from build123d import *

# Parameters (mm, degrees)
F0_W     = 112
F0_H     = 120
F1_DEPTH = 20
F2_DEPTH = 60
F3_SIZE2 = 34.641006
F3_SIZE  = 59.99999
F4_SIZE2 = 34.641006
F4_SIZE  = 59.99999
F5_R     = 20
F7_R     = 30
F8_R     = 10


# Not quite as in the source:
# - a fillet or chamfer is up to 0.001 mm smaller than in the source, because OpenCascade refuses the exact size


with BuildPart() as f1:
    # F0 (on Top) → F1 (new body)
    with BuildSketch(Plane.XY):
        with Locations((0.0172033906, -34.0157587473)):
            Rectangle(F0_W, F0_H)
    extrude(amount=F1_DEPTH)


with BuildPart() as f2:
    # F2 (new): a face of the model
    f2_faces = [f1.part.faces().sort_by_distance(p)[0] for p in [
        (0.0172033906, -34.0157587473, 20),
    ]]
    extrude(f2_faces, amount=F2_DEPTH)

    # F3 (size 60 and 34.6410161514 in the source; OpenCascade refuses exactly that, so slightly less here)
    f3_edges = [f2.edges().sort_by_distance(p)[0] for p in [
        (56.017203, -34.015759, 80),
    ]]
    f3_side = f2.faces().sort_by_distance((56.017203, -34.015759, 50))[0]
    chamfer(f3_edges, length=F3_SIZE, length2=F3_SIZE2, reference=f3_side)

    # F4 (size 60 and 34.6410161514 in the source; OpenCascade refuses exactly that, so slightly less here)
    f4_edges = [f2.edges().sort_by_distance(p)[0] for p in [
        (-55.982797, -34.015759, 80),
    ]]
    f4_side = f2.faces().sort_by_distance((-55.982797, -34.015759, 50))[0]
    chamfer(f4_edges, length=F4_SIZE, length2=F4_SIZE2, reference=f4_side)

    # F5
    f5_edges = [f2.edges().sort_by_distance(p)[0] for p in [
        (21.376197, -34.015759, 80),
        (-21.341791, -34.015759, 80),
    ]]
    fillet(f5_edges, radius=F5_R)


with BuildPart() as f1_1:
    add(f1.part)

    # F6: union F2
    add(f2.part)

    # F7
    f7_edges = [f1_1.edges().sort_by_distance(p)[0] for p in [
        (-55.982797, -34.015759, 20),
        (56.017203, -34.015759, 20),
    ]]
    fillet(f7_edges, radius=F7_R)

    # F8
    f8_edges = [f1_1.edges().sort_by_distance(p)[0] for p in [
        (-39.539426, -94.015759, 48.480766),
        (-55.982797, -94.015759, 5.980768),
        (-39.539426, 25.984241, 48.480766),
        (-55.982797, 25.984241, 5.980768),
    ]]
    fillet(f8_edges, radius=F8_R)


solid = f1_1.part
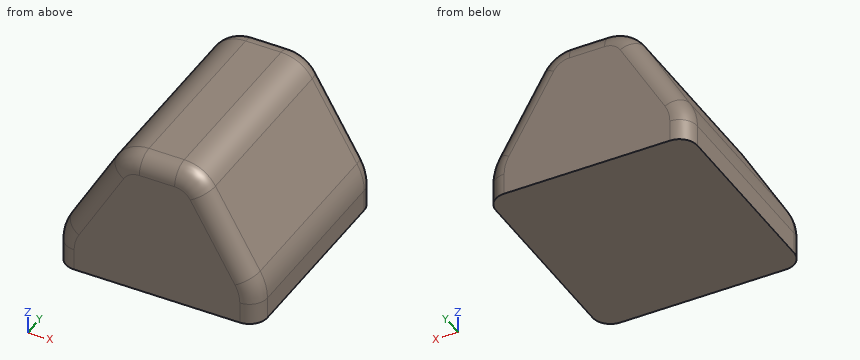
Input: part model. Units: mm. Frame: model coordinates. Give positions to 0.01 mm unless a question says otherwise; leave off trailing zeros. Loops run counter-clockwise (first coordinate to the right, second up) from the corner with the lowest first, then second, coordinate; pieces in that order, holes last. Notation, with made-up numbers: M -9,30.5 L 30,30.5 A31 ccw 30,59.5 Z; hole C 14,8.5 d7. An arc over 180 degrees is marked long. Use one line per item in the form item = value.
1. Line query: L1, parallel to Z at x = 10, y = -26.5; L2, parallel to Y at x = -0.5, z = 73; L3, parallel to Z at x = -44.5, y = -42. Output: solid intervals per line, ascending.
Numbers:
L1 = 0 to 80
L2 = -93.56 to 25.52
L3 = 0 to 39.89
2. Section query A-A, the plane y = -70.5. Return the cut outline in (x, z), and give its area (3 significant figures).
Numbers:
outline = M -55.98,0 L 56.02,0 L 56.02,11.96 A30 ccw 52,26.96 L 27.15,70 A20 ccw 9.83,80 L -9.79,80 A20 ccw -27.12,70 L -51.96,26.96 A30 ccw -55.98,11.96 Z
area = 6,830 mm²
3. First-contact query: pin 1 (3 mm diameter, centred on y = -57, z = 21, fed in from +X); pin 2 (6 mm diameter, centred on x = -32.5, z = 47, fed in from +Y); pin 3 (6 mm diameter, centred on y = 6.5, z = 27.5, fed in from +X). Flat tips, straight axial feed; report the tip coordinate or a pass-through.
Numbers:
pin_1 = 55.05
pin_2 = 25.98
pin_3 = 53.27
